Design review of the part built by this model. Coordinates are the model's own, in mm. A direction names the side the tool comes from. Round coordinates to 2 decimals unless told otherwise and drop trailing zeros. Write each loop counter-clockwise with the first axis right and the second up, starting at its lowest first coordinate (ties: lowest second). Pieces come first, ordered by that corner, then holes. Notation, with made-up numbers: (81.5, -25.5) -> (124.5, -25.5) arc R19 cw to (124.5, -13.5) -> close; hole circle Ø3 at (-5.5, 79.25). An arc over 180 degrees is marked (long way). One line per question, with ' | ' between items. Start each with the question number.
1) Mouldability with a two-part tool opening along Y and no side actions: class faces 1 (the flat face through (-33.325, 27.294, -15.042)), 2 (the flat face through (28, 18, 12)), 3 (the cylindrical face through (1.041, 31.932, 14.958)) as +Y half, -Y half, draft (parallel to the pull), parting line (faces both ways), or undercut.
2) Consider section C-C (x = -34). Give the boundary of the cut face in (y, z), then the cut area to 3 significant figures.
3) For probe 1 along Z at (x, y) = (34, 1.4); probe 2 along X at (y, z) = (17.5, -7.5); probe 3 along Z at (x, y) = (-25, 10), list the stretches that pass through material, from the lowest coordinate up.
4) Insertion check: pin 1 Ø18.5 at (x, y) = (0, 24) entering from -Z; pin 2 Ø7 at (x, z) = (-33, 4.5) entering from +Y; pin 3 Ø7.5 at (x, y) = (37.5, 22) entering from +Z; pin 4 Ø6 at (x, z) = (-34, 0) entering from +Y. Each pin has a flat end and moves straight along its axis. Give the tip position at first contact, or say it passes through.
5) Consider section D-D (z = 17). Give the boundary of the cut face in (x, y), then the cut area to 3 significant figures.
6) For faces 4 (the flat face through (-1, 6, -21)), 5 (the flat face through (-0.2, 42, -8.2)), 6 (the flat face through (-34, 6, -6)), list the 3-axis set-ups (+Z, -Z, +X, -X, +Y, -Y) from which the entire face can be reached by the end or side of a thin tool; tool diameter is ignored.
7) Consider section A-A (x = 0). Give the boundary of the cut face in (y, z).
8) Consider section B-B (z = 0). Give the boundary of the cut face in (x, y), then the cut area to 3 significant figures.
```python
from build123d import *

# Parameters (mm, degrees)
SCHIZZO1_W                   = 92
SCHIZZO1_H                   = 48
SCHIZZO1_W_2                 = 30
SCHIZZO1_H_2                 = 24
ESTRUSIONE_ESTRUSIONE1_DEPTH = 6
SCHIZZO2_W                   = 42
SCHIZZO2_H                   = 36
SCHIZZO2_W_2                 = 30
SCHIZZO2_H_2                 = 24
ESTRUSIONE_ESTRUSIONE2_DEPTH = 36
SCHIZZO3_W                   = 42
SCHIZZO3_H                   = 36
ESTRUSIONE_ESTRUSIONE3_DEPTH = 6
ESTRUSIONE_ESTRUSIONE4_DEPTH = 6
FORO_16_0_16_1_D             = 16
FORO_16_0_16_2_D             = 16
FORO_10_0_10_1_D             = 10


with BuildPart() as part:
    # Schizzo1 → Estrusione-Estrusione1 (new body)
    with BuildSketch(Plane(origin=(0, 0, 0), x_dir=(1, 0, 0), z_dir=(0, 1, 0))):
        Rectangle(SCHIZZO1_W, SCHIZZO1_H)
        Rectangle(SCHIZZO1_W_2, SCHIZZO1_H_2, mode=Mode.SUBTRACT)
    extrude(amount=ESTRUSIONE_ESTRUSIONE1_DEPTH)

    # Schizzo2 → Estrusione-Estrusione2 (add)
    with BuildSketch(Plane(origin=(0, 6, 0), x_dir=(1, 0, 0), z_dir=(0, 1, 0))):
        Rectangle(SCHIZZO2_W, SCHIZZO2_H)
        Rectangle(SCHIZZO2_W_2, SCHIZZO2_H_2, mode=Mode.SUBTRACT)
    extrude(amount=ESTRUSIONE_ESTRUSIONE2_DEPTH)

    # Schizzo3 → Estrusione-Estrusione3 (add)
    with BuildSketch(Plane(origin=(0, 42, 0), x_dir=(1, 0, 0), z_dir=(0, 1, 0))):
        Rectangle(SCHIZZO3_W, SCHIZZO3_H)
    extrude(amount=ESTRUSIONE_ESTRUSIONE3_DEPTH)

    # Schizzo4 → Estrusione-Estrusione4 (add)
    with BuildSketch(Plane.XY.offset(18)):
        Polygon((-21, 48), (-46, 6), (-21, 6), align=None)
        Polygon((21, 48), (46, 6), (21, 6), align=None)
    estrusione_estrusione4 = extrude(amount=-ESTRUSIONE_ESTRUSIONE4_DEPTH)

    # Specchia1: Estrusione-Estrusione4 across plane
    add(estrusione_estrusione4.mirror(Plane.XY))

    # Foro Ø16.0 (16)-1 (through all)
    with Locations(Plane.XY.offset(18)):
        with Locations((0, 24)):
            Hole(FORO_16_0_16_1_D / 2)

    # Foro Ø16.0 (16)-2 (through all)
    with Locations(Plane(origin=(0, 48, 0), x_dir=(1, 0, 0), z_dir=(0, 1, 0))):
        with Locations((0, 0)):
            Hole(FORO_16_0_16_2_D / 2)

    # Foro Ø10.0 (10)-1 (through all)
    with Locations(Plane(origin=(0, 6, 0), x_dir=(1, 0, 0), z_dir=(0, 1, 0))):
        with Locations((-34, 0), (34, 0)):
            Hole(FORO_10_0_10_1_D / 2)


solid = part.part
```
From the geometry:
1) face 1: +Y half | face 2: draft | face 3: undercut
2) outline: (0, -24) -> (6, -24) -> (6, -18) -> (26.16, -18) -> (26.16, -12) -> (6, -12) -> (6, -5) -> (0, -5) -> close; (0, 5) -> (6, 5) -> (6, 12) -> (26.16, 12) -> (26.16, 18) -> (6, 18) -> (6, 24) -> (0, 24) -> close | area: 470 mm2
3) probe 1: z = -24 to -5, 5 to 24 | probe 2: x = -21 to -15, 15 to 21 | probe 3: z = -18 to -12, 12 to 18
4) pin 1: stops at z = -18 | pin 2: stops at y = 6 | pin 3: stops at z = 18 | pin 4: passes through
5) outline: (-46, 0) -> (46, 0) -> (46, 6) -> (21, 48) -> (-21, 48) -> (-46, 6) -> close; hole circle Ø16 at (0, 24) | area: 3,160 mm2
6) face 4: -Z, +X, -X, +Y | face 5: -Y | face 6: -X, +Y
7) outline: (0, -24) -> (6, -24) -> (6, -18) -> (16, -18) -> (16, -12) -> (0, -12) -> close; (0, 12) -> (16, 12) -> (16, 18) -> (6, 18) -> (6, 24) -> (0, 24) -> close; (32, -18) -> (48, -18) -> (48, -8) -> (42, -8) -> (42, -12) -> (32, -12) -> close; (32, 12) -> (42, 12) -> (42, 8) -> (48, 8) -> (48, 18) -> (32, 18) -> close
8) outline: (-46, 0) -> (-39, 0) -> (-39, 6) -> (-46, 6) -> close; (-29, 0) -> (-15, 0) -> (-15, 42) -> (-8, 42) -> (-8, 48) -> (-21, 48) -> (-21, 6) -> (-29, 6) -> close; (8, 42) -> (15, 42) -> (15, 0) -> (29, 0) -> (29, 6) -> (21, 6) -> (21, 48) -> (8, 48) -> close; (39, 0) -> (46, 0) -> (46, 6) -> (39, 6) -> close | area: 840 mm2
